Geometry: final body of the model. Coordinates: model frame, mm. A direction names the side the tool comes from. Give positions to 0.01 mm unless a question says otherwise; leave off trailing zeros. Write each loop counter-clockwise with the first axis right and the second up, starting at its lowest first coordinate (ties: lowest second). Pieces come first, ordered by that corner, then holes.
Q1. Reachability of faces 4 (the face through (11.555, 19, 5)), 5 (the face through (28, 9, 1)), 6 (the face through (-29, -11, 1)) from +Z, -Z, +X, -X, +Y, -Y: full face, straight path, thin tool, end or side. Return the list, or none.
Q2. Cut plane C-C on y = 4. Return the cut outline in (x, z), plus the area to 3 significant figures.
Q3. Pin query (flat end, axial travel): pin 1 (1.8 mm diameter, centred on y = 18.5, z = 6, fed in from -X); pin 2 (2 mm diameter, centred on y = 10.5, z = 3.5, fed in from +X); pin 3 (2.5 mm diameter, centred on x = -30, y = 5, fed in from +Z). Return the tip coordinate at first contact, or that it passes through.
Q4. Cut plane D-D on z = 1. Count the separate pieces of the cut face and the enclosed holes in it, plus the area to 3 significant figures.
Q5. Cut plane B-B on x = 15.5. Return the cut outline in (y, z), plus the area to 3 significant figures.
Q6. Cut plane A-A on z = 6.75. Return the cut outline in (x, y), plus the area to 3 significant figures.
Q7. Line query: L1, parallel to X at y = -4, z = 1.25; L2, parallel to Y at x = 6, z = 8.75; L3, parallel to X at y = 6, z = 8. Output: solid intervals per line, ascending.
Q8. Draft query along X for faces 1 (the face through (0, 18, 10.2)), 2 (the face through (-32.2, 0, 1)), 3 (the face through (27.2, 0, 5)). Return one class per face: pulls with the +X half, pulls with the -X half, needs draft (parallel to the pull), parting line crosses it, or undercut.
```python
from build123d import *

# Parameters (mm, degrees)
BOSS_EXTRUDE1_DEPTH = 10.2
CUT_EXTRUDE1_DEPTH  = 8
BOSS_EXTRUDE2_DEPTH = 2.2
CUT_EXTRUDE2_DEPTH  = 2.2
SKETCH6_W           = 10.84
SKETCH6_H           = 6.17
CUT_EXTRUDE3_DEPTH  = 46
SKETCH8_W           = 6.99
SKETCH8_H           = 5.66
CUT_EXTRUDE4_DEPTH  = 29


with BuildPart() as part:
    # Sketch1 → Boss-Extrude1 (new body)
    with BuildSketch(Plane.XY):
        with BuildLine():
            Line((23.2, -19.7), (-23.2, -19.7))
            ThreePointArc((-23.2, -19.7), (-26.028427125, -18.528427125), (-27.2, -15.7))
            Line((-27.2, -15.7), (-27.2, 15.7))
            ThreePointArc((-27.2, 15.7), (-26.028427125, 18.528427125), (-23.2, 19.7))
            Line((-23.2, 19.7), (23.2, 19.7))
            ThreePointArc((23.2, 19.7), (26.028427125, 18.528427125), (27.2, 15.7))
            Line((27.2, 15.7), (27.2, -15.7))
            ThreePointArc((27.2, -15.7), (26.028427125, -18.528427125), (23.2, -19.7))
        make_face()
    extrude(amount=BOSS_EXTRUDE1_DEPTH)

    # Sketch2 → Cut-Extrude1 (cut)
    with BuildSketch(Plane.XY.offset(10.2)):
        with BuildLine():
            Line((21, -17.5), (-21, -17.5))
            ThreePointArc((-21, -17.5), (-23.828427125, -16.328427125), (-25, -13.5))
            Line((-25, -13.5), (-25, 13.5))
            ThreePointArc((-25, 13.5), (-23.828427125, 16.328427125), (-21, 17.5))
            Line((-21, 17.5), (21, 17.5))
            ThreePointArc((21, 17.5), (23.828427125, 16.328427125), (25, 13.5))
            Line((25, 13.5), (25, -13.5))
            ThreePointArc((25, -13.5), (23.828427125, -16.328427125), (21, -17.5))
        make_face()
    extrude(amount=-CUT_EXTRUDE1_DEPTH, mode=Mode.SUBTRACT)

    # Sketch4 → Boss-Extrude2 (add)
    with BuildSketch(Plane.XY.offset(2.2)):
        with BuildLine():
            Line((27.2, -11), (31.2, -11))
            ThreePointArc((31.2, -11), (31.907106781, -10.707106781), (32.2, -10))
            Line((32.2, -10), (32.2, 10))
            ThreePointArc((32.2, 10), (31.907106781, 10.707106781), (31.2, 11))
            Line((31.2, 11), (27.2, 11))
            Line((27.2, 11), (27.2, -11))
        make_face()
        with BuildLine():
            Line((-27.2, 11), (-27.2, -11))
            Line((-27.2, -11), (-31.2, -11))
            ThreePointArc((-31.2, -11), (-31.907106781, -10.707106781), (-32.2, -10))
            Line((-32.2, -10), (-32.2, 10))
            ThreePointArc((-32.2, 10), (-31.907106781, 10.707106781), (-31.2, 11))
            Line((-31.2, 11), (-27.2, 11))
        make_face()
    extrude(amount=-BOSS_EXTRUDE2_DEPTH)

    # Sketch5 → Cut-Extrude2 (cut)
    with BuildSketch(Plane.XY.offset(2.2)):
        with BuildLine():
            Line((27.2, -9), (29.2, -9))
            ThreePointArc((29.2, -9), (29.907106781, -8.707106781), (30.2, -8))
            Line((30.2, -8), (30.2, 8))
            ThreePointArc((30.2, 8), (29.907106781, 8.707106781), (29.2, 9))
            Line((29.2, 9), (27.2, 9))
            Line((27.2, 9), (27.2, -9))
        make_face()
        with BuildLine():
            Line((-27.2, -9), (-27.2, 9))
            Line((-27.2, 9), (-29.2, 9))
            ThreePointArc((-29.2, 9), (-29.907106781, 8.707106781), (-30.2, 8))
            Line((-30.2, 8), (-30.2, -8))
            ThreePointArc((-30.2, -8), (-29.907106781, -8.707106781), (-29.2, -9))
            Line((-29.2, -9), (-27.2, -9))
        make_face()
    extrude(amount=-CUT_EXTRUDE2_DEPTH, mode=Mode.SUBTRACT)

    # Sketch6 → Cut-Extrude3 (cut)
    with BuildSketch(Plane(origin=(0, 0, 0), x_dir=(1, 0, 0), z_dir=(0, 1, 0))):
        with Locations((-14.720967814, -5.285)):
            Rectangle(SKETCH6_W, SKETCH6_H)
    extrude(amount=CUT_EXTRUDE3_DEPTH, mode=Mode.SUBTRACT)

    # Sketch8 → Cut-Extrude4 (cut)
    with BuildSketch(Plane(origin=(0, 0, 0), x_dir=(1, 0, 0), z_dir=(0, 1, 0))):
        with Locations((8.059896405, -5.03)):
            Rectangle(SKETCH8_W, SKETCH8_H)
    extrude(amount=CUT_EXTRUDE4_DEPTH, mode=Mode.SUBTRACT)


solid = part.part
```
Data:
1. face 4: +Y
1. face 5: +Z, -Z
1. face 6: +Z, -Z, -X, -Y
2. outline: (-32.2, 0) - (-30.2, 0) - (-30.2, 2.2) - (-32.2, 2.2) - close; (-27.2, 0) - (27.2, 0) - (27.2, 10.2) - (25, 10.2) - (25, 2.2) - (-25, 2.2) - (-25, 10.2) - (-27.2, 10.2) - close; (30.2, 0) - (32.2, 0) - (32.2, 2.2) - (30.2, 2.2) - close
2. area: 164 mm2
3. pin 1: stops at x = -26.72
3. pin 2: stops at x = 27.2
3. pin 3: stops at z = 2.2
4. separate pieces: 1
4. enclosed holes: 2
4. area: 2,240 mm2
5. outline: (-19.7, 0) - (19.7, 0) - (19.7, 10.2) - (17.5, 10.2) - (17.5, 2.2) - (-17.5, 2.2) - (-17.5, 10.2) - (-19.7, 10.2) - close
5. area: 122 mm2
6. outline: (-27.2, -15.7) arc R4 ccw to (-23.2, -19.7) - (23.2, -19.7) arc R4 ccw to (27.2, -15.7) - (27.2, 15.7) arc R4 ccw to (23.2, 19.7) - (11.55, 19.7) - (11.55, 17.5) - (21, 17.5) arc R4 cw to (25, 13.5) - (25, -13.5) arc R4 cw to (21, -17.5) - (-21, -17.5) arc R4 cw to (-25, -13.5) - (-25, 13.5) arc R4 cw to (-21, 17.5) - (-20.14, 17.5) - (-20.14, 19.7) - (-23.2, 19.7) arc R4 ccw to (-27.2, 15.7) - close; (-9.3, 17.5) - (4.56, 17.5) - (4.56, 19.7) - (-9.3, 19.7) - close
6. area: 354 mm2
7. L1: x = -32.2 to -30.2, -27.2 to 27.2, 30.2 to 32.2
7. L2: y = -19.7 to -17.5, 17.5 to 19.7
7. L3: x = -27.2 to -25, 25 to 27.2
8. face 1: needs draft
8. face 2: pulls with the -X half
8. face 3: undercut
